```python
from build123d import *

# Parameters (mm, degrees)
SKETCH_W  = 200
SKETCH_H  = 65
SKETCH_R  = 2
PAD_DEPTH = 10
FILLET_R  = 3


with BuildPart() as part:
    # Sketch → Pad (new body)
    with BuildSketch(Plane.XY):
        with Locations((100, 32.5)):
            Rectangle(SKETCH_W, SKETCH_H)
        with Locations((30, 50)):
            Circle(SKETCH_R, mode=Mode.SUBTRACT)
        with Locations((30, 15)):
            Circle(SKETCH_R, mode=Mode.SUBTRACT)
        with Locations((170, 50)):
            Circle(SKETCH_R, mode=Mode.SUBTRACT)
        with Locations((170, 15)):
            Circle(SKETCH_R, mode=Mode.SUBTRACT)
        with Locations((50, 50)):
            Circle(SKETCH_R, mode=Mode.SUBTRACT)
        with Locations((50, 15)):
            Circle(SKETCH_R, mode=Mode.SUBTRACT)
        with Locations((150, 50)):
            Circle(SKETCH_R, mode=Mode.SUBTRACT)
        with Locations((150, 15)):
            Circle(SKETCH_R, mode=Mode.SUBTRACT)
        with Locations((70, 50)):
            Circle(SKETCH_R, mode=Mode.SUBTRACT)
        with Locations((70, 15)):
            Circle(SKETCH_R, mode=Mode.SUBTRACT)
        with Locations((130, 15)):
            Circle(SKETCH_R, mode=Mode.SUBTRACT)
        with Locations((130, 50)):
            Circle(SKETCH_R, mode=Mode.SUBTRACT)
    extrude(amount=PAD_DEPTH)

    # Fillet
    fillet_edges = [part.edges().sort_by_distance(p)[0] for p in [
        (200, 0, 5),
        (0, 0, 5),
        (200, 65, 5),
        (0, 65, 5),
    ]]
    fillet(fillet_edges, radius=FILLET_R)


solid = part.part
```
Verification items for the finished model (mm, model axes). Coordinates: 2 decimals unless noted, no trailing zeros. Order: outer loops, then holes, each group sorted by start corner. A loop starts at its lowest first (then second) coordinate and runs counter-clockwise, first axis right, second up. Notation, with made-up numbers: (42.25, 37.5) -> (101.25, 37.5) arc R6 ccw to (101.25, 41.5) -> close; hole circle Ø1 at (-26.5, -22.75). An arc over 180 degrees is marked (long way). Put each result on its own line as item: value. Start each with the question number.
1) Cross-section at B-B (x = 70). Enter the section's corners in (y, z), plus the area to 3 significant figures.
2) Cross-section at A-A (y = 15). Enter the section's corners in (x, z), plus the area to 3 significant figures.
3) Material ranges on L1, parallel to Y at x = 150, z = 3.5; L2, parallel to Y at x = 49.5, z = 1.25, recorded low to high.
4) Release check for a two-part mould opening along X. For faces 1 (the cylindrical face through (128.4, 48.8, 4.9)), 2 (the flat face through (99, 0, 5)), 3 (the flat face through (0, 32, 5)) record: pulls with the +X half, pulls with the -X half, needs draft (parallel to the pull), parting line crosses it, or undercut.
5) Go/stop test with a flat-tipped pin: pin 1 (3 mm diameter, centred on x = 130, y = 15, fed in from -Z). Record where the tip stops, or that it passes through.
Geometry check:
1. outline: (0, 0) -> (13, 0) -> (13, 10) -> (0, 10) -> close; (17, 0) -> (48, 0) -> (48, 10) -> (17, 10) -> close; (52, 0) -> (65, 0) -> (65, 10) -> (52, 10) -> close
1. area: 570 mm^2
2. outline: (0, 0) -> (28, 0) -> (28, 10) -> (0, 10) -> close; (32, 0) -> (48, 0) -> (48, 10) -> (32, 10) -> close; (52, 0) -> (68, 0) -> (68, 10) -> (52, 10) -> close; (72, 0) -> (128, 0) -> (128, 10) -> (72, 10) -> close; (132, 0) -> (148, 0) -> (148, 10) -> (132, 10) -> close; (152, 0) -> (168, 0) -> (168, 10) -> (152, 10) -> close; (172, 0) -> (200, 0) -> (200, 10) -> (172, 10) -> close
2. area: 1,760 mm^2
3. L1: y = 0 to 13, 17 to 48, 52 to 65
3. L2: y = 0 to 13.06, 16.94 to 48.06, 51.94 to 65
4. face 1: undercut
4. face 2: needs draft
4. face 3: pulls with the -X half
5. pin 1: passes through
